from build123d import *

# Parameters (mm, degrees)
ESQUISSE1_R                  = 5
BOSS_EXTRU_1_DEPTH           = 2.9
BOSS_EXTRU_2_DEPTH           = 3
BOSS_EXTRU_3_DEPTH           = 2
ESQUISSE4_R                  = 0.8
ENL_V_MAT_EXTRU_1_DEPTH      = 6.9
ESQUISSE5_R                  = 0.8
ENL_V_MAT_EXTRU_2_DEPTH      = 6.9
R_P_TITION_CIRCULAIRE1_COUNT = 2
ESQUISSE6_R                  = 3
ENL_V_MAT_EXTRU_3_DEPTH      = 1.4
ESQUISSE7_R                  = 1.4
ENL_V_MAT_EXTRU_4_DEPTH      = 5.5


with BuildPart() as part:
    # Esquisse1 → Boss.-Extru.1 (new body)
    with BuildSketch(Plane.XY):
        Circle(ESQUISSE1_R)
        Polygon((2.011577371, -1.550856692), (2.011577371, -2.011577371), (1.550856692, -2.011577371), (1.541643286, -2.018647066), (1.4224, -2.463669069), (0.977377998, -2.344425783), (0.966648759, -2.348869979), (0.73628842, -2.747865791), (0.337292608, -2.517505451), (0.325778716, -2.519021284), (0, -2.8448), (-0.325778716, -2.519021284), (-0.337292608, -2.517505451), (-0.73628842, -2.747865791), (-0.966648759, -2.348869979), (-0.977377998, -2.344425783), (-1.4224, -2.463669069), (-1.541643286, -2.018647066), (-1.550856692, -2.011577371), (-2.011577371, -2.011577371), (-2.011577371, -1.550856692), (-2.018647066, -1.541643286), (-2.463669069, -1.4224), (-2.344425783, -0.977377998), (-2.348869979, -0.966648759), (-2.747865791, -0.73628842), (-2.517505451, -0.337292608), (-2.519021284, -0.325778716), (-2.8448, 0), (-2.519021284, 0.325778716), (-2.517505451, 0.337292608), (-2.747865791, 0.73628842), (-2.348869979, 0.966648759), (-2.344425783, 0.977377998), (-2.463669069, 1.4224), (-2.018647066, 1.541643286), (-2.011577371, 1.550856692), (-2.011577371, 2.011577371), (-1.550856692, 2.011577371), (-1.541643286, 2.018647066), (-1.4224, 2.463669069), (-0.977377998, 2.344425783), (-0.966648759, 2.348869979), (-0.73628842, 2.747865791), (-0.337292608, 2.517505451), (-0.325778716, 2.519021284), (0, 2.8448), (0.325778716, 2.519021284), (0.337292608, 2.517505451), (0.73628842, 2.747865791), (0.966648759, 2.348869979), (0.977377998, 2.344425783), (1.4224, 2.463669069), (1.541643286, 2.018647066), (1.550856692, 2.011577371), (2.011577371, 2.011577371), (2.011577371, 1.550856692), (2.018647066, 1.541643286), (2.463669069, 1.4224), (2.344425783, 0.977377998), (2.348869979, 0.966648759), (2.747865791, 0.73628842), (2.517505451, 0.337292608), (2.519021284, 0.325778716), (2.8448, 0), (2.519021284, -0.325778716), (2.517505451, -0.337292608), (2.747865791, -0.73628842), (2.348869979, -0.966648759), (2.344425783, -0.977377998), (2.463669069, -1.4224), (2.018647066, -1.541643286), align=None, mode=Mode.SUBTRACT)
    extrude(amount=BOSS_EXTRU_1_DEPTH)

    # Esquisse2 → Boss.-Extru.2 (add)
    with BuildSketch(Plane.XY.offset(2.9)):
        with BuildLine():
            Line((-16, 5.8), (16, 5.8))
            ThreePointArc((16, 5.8), (21.8, 0), (16, -5.8))
            Line((16, -5.8), (-16, -5.8))
            ThreePointArc((-16, -5.8), (-21.8, 0), (-16, 5.8))
        make_face()
    extrude(amount=BOSS_EXTRU_2_DEPTH)

    # Esquisse3 → Boss.-Extru.3 (add)
    with BuildSketch(Plane.XY.offset(5.9)):
        with BuildLine():
            Line((5.8, 16), (5.8, -16))
            ThreePointArc((5.8, -16), (0, -21.8), (-5.8, -16))
            Line((-5.8, -16), (-5.8, 16))
            ThreePointArc((-5.8, 16), (0, 21.8), (5.8, 16))
        make_face()
    extrude(amount=-BOSS_EXTRU_3_DEPTH)

    # Esquisse4 → Enlèv. mat.-Extru.1 (cut, through all)
    with BuildSketch(Plane.XY.offset(5.9)):
        with Locations((-10, 0)):
            Circle(ESQUISSE4_R)
        with Locations((-13, 0)):
            Circle(ESQUISSE4_R)
        with Locations((-16, 0)):
            Circle(ESQUISSE4_R)
        with Locations((-19, 0)):
            Circle(ESQUISSE4_R)
    enl_v_mat_extru_1 = extrude(amount=-ENL_V_MAT_EXTRU_1_DEPTH, mode=Mode.SUBTRACT)

    # Esquisse5 → Enlèv. mat.-Extru.2 (cut, through all)
    with BuildSketch(Plane.XY.offset(5.9)):
        with Locations((0, 12)):
            Circle(ESQUISSE5_R)
        with Locations((0, 15)):
            Circle(ESQUISSE5_R)
        with Locations((0, 18)):
            Circle(ESQUISSE5_R)
    enl_v_mat_extru_2 = extrude(amount=-ENL_V_MAT_EXTRU_2_DEPTH, mode=Mode.SUBTRACT)

    # Répétition circulaire1: Enlèv. mat.-Extru.1, Enlèv. mat.-Extru.2 ×2 about axis
    r_p_tition_circulaire1_axis = Axis((0, 0, 0), (0, 0, 1))
    for i in range(1, R_P_TITION_CIRCULAIRE1_COUNT):
        add(enl_v_mat_extru_1.rotate(r_p_tition_circulaire1_axis, i * 360 / R_P_TITION_CIRCULAIRE1_COUNT), mode=Mode.SUBTRACT)
        add(enl_v_mat_extru_2.rotate(r_p_tition_circulaire1_axis, i * 360 / R_P_TITION_CIRCULAIRE1_COUNT), mode=Mode.SUBTRACT)

    # Esquisse6 → Enlèv. mat.-Extru.3 (cut)
    with BuildSketch(Plane.XY.offset(5.9)):
        Circle(ESQUISSE6_R)
    extrude(amount=-ENL_V_MAT_EXTRU_3_DEPTH, mode=Mode.SUBTRACT)

    # Esquisse7 → Enlèv. mat.-Extru.4 (cut, through all)
    with BuildSketch(Plane.XY.offset(4.5)):
        Circle(ESQUISSE7_R)
    extrude(amount=-ENL_V_MAT_EXTRU_4_DEPTH, mode=Mode.SUBTRACT)


solid = part.part
Check sheet for the modelled part. Datum: model origin and axes. Units: mm. A direction names the side the tool comes from. Round coordinates to 2 decimals unless told otherwise and drop trailing zeros. Loops run counter-clockwise (first coordinate to the right, second up) from the corner with the lowest first, then second, coordinate; pieces in that order, holes last.
1. Scan lines: probe 1 along X at (y, z) = (-15, 5.4); probe 2 along Z at (x, y) = (-1, 14). Record each from-to range of solid material in increasing order.
2. Gauge pin test, flat ends, axial feed: pin 1 Ø3 at (x, y) = (9.5, 5.5) entering from -Z; pin 2 Ø3.5 at (x, z) = (6.5, 4.5) entering from +Y; pin 3 Ø1 at (x, y) = (16, 0) entering from +Z; pin 4 Ø1.5 at (x, z) = (13, 2.5) entering from -Y. Record the tip position at first contact, or that the pin passes through.
3. Set-up check for faces 4 (the flat face through (1.3, 1.3, 2.9)), 5 (the cylindrical face through (-3, 0, 5)), 6 (the flat face through (-5.8, -11, 5)), 7 (the flat face through (2.2, -2.2, 0)), 8 (the flat face through (5.8, -11, 5)): record each of +Z, -Z, +X, -X, +Y, -Y from which the full face is reachable in a straight line by a thin tool's end or side.
4. Sectioned sample at D-D on x = 11.5. Record the boundary of the cut face in (y, z).
5. Sectioned sample at B-B on x = -13. Record the boundary of the cut face in (y, z).
6. Mould release check, pull along Y, two halves, no side actions. Record for faces 1 (the flat face through (0, -5, 5.9)), 2 (the cylindrical face through (0.1, -21.8, 4.9)), 3 (the cylindrical face through (-1.4, 0.06, 3.71)): released by +Y, released by -Y, zero draft, split by the parting line, or undercut.
7. Sectioned sample at C-C on y = 7. Record the boundary of the cut face in (x, z).
8. Sectioned sample at A-A on y = 15. Record the boundary of the cut face in (x, z).
Recorded:
1. probe 1: x = -5.8 to -0.8, 0.8 to 5.8
1. probe 2: z = 3.9 to 5.9
2. pin 1: stops at z = 2.9
2. pin 2: stops at y = 19.33
2. pin 3: passes through
2. pin 4: stops at y = -5.8
3. face 4: -Z
3. face 5: +Z
3. face 6: +Z, -Z, -X, -Y
3. face 7: -Z, +X, -X, +Y, -Y
3. face 8: +Z, -Z, +X, -Y
4. outline: (-5.8, 2.9) - (5.8, 2.9) - (5.8, 5.9) - (-5.8, 5.9) - close
5. outline: (-5.8, 2.9) - (-0.8, 2.9) - (-0.8, 5.9) - (-5.8, 5.9) - close; (0.8, 2.9) - (5.8, 2.9) - (5.8, 5.9) - (0.8, 5.9) - close
6. face 1: zero draft
6. face 2: released by -Y
6. face 3: undercut
7. outline: (-5.8, 3.9) - (5.8, 3.9) - (5.8, 5.9) - (-5.8, 5.9) - close
8. outline: (-5.8, 3.9) - (-0.8, 3.9) - (-0.8, 5.9) - (-5.8, 5.9) - close; (0.8, 3.9) - (5.8, 3.9) - (5.8, 5.9) - (0.8, 5.9) - close
